```python
from build123d import *

# Parameters (mm, degrees)
SKETCH1_W            = 24
SKETCH1_H            = 24
BOSS_EXTRUDE1_DEPTH  = 3
SKETCH2_W            = 16.6
SKETCH2_H            = 12
BOSS_EXTRUDE2_DEPTH  = 8
CUT_EXTRUDE1_DEPTH   = 21.223748416
CUT_EXTRUDE2_REACH   = 30.26
SKETCH4_R            = 1.6
CUT_EXTRUDE3_DEPTH   = 1.3
FILLET3_R            = 6
CHAMFER3_SIZE        = 3
FILLET4_R            = 3
FILLET6_R            = 1
SKETCH9_R            = 1.6
CUT_EXTRUDE5_DEPTH   = 19.761663039
FILLET8_R            = 3
FILLET9_R            = 0.5
CUT_EXTRUDE6_START   = -1
CUT_EXTRUDE6_DEPTH   = 20.761663103
MIRROR2_START        = -1
MIRROR2_COPY_1_DEPTH = 20.761663103


with BuildPart() as part:
    # Sketch1 → Boss-Extrude1 (new body)
    with BuildSketch(Plane(origin=(0, 0, 0), x_dir=(1, 0, 0), z_dir=(0, 1, 0))):
        Rectangle(SKETCH1_W, SKETCH1_H)
    extrude(amount=BOSS_EXTRUDE1_DEPTH)

    # Sketch2 → Boss-Extrude2 (add)
    with BuildSketch(Plane(origin=(0, 3, 0), x_dir=(1, 0, 0), z_dir=(0, 1, 0))):
        with Locations((-2.8, 0)):
            Rectangle(SKETCH2_W, SKETCH2_H)
    extrude(amount=BOSS_EXTRUDE2_DEPTH)

    # Sketch3 → Cut-Extrude1 (cut, through all)
    with BuildSketch(Plane(origin=(0, 11, 0), x_dir=(1, 0, 0), z_dir=(0, 1, 0))):
        with BuildLine():
            Line((-1.9, 1.774823935), (-1.9, -1.774823935))
            ThreePointArc((-1.9, -1.774823935), (2.6, 0), (-1.9, 1.774823935))
        make_face()
    extrude(amount=-CUT_EXTRUDE1_DEPTH, mode=Mode.SUBTRACT)

    # Sketch4 → Cut-Extrude2 (cut, up to next)
    with BuildSketch(Plane.ZY.offset(11.1), mode=Mode.PRIVATE) as cut_extrude2_sk1:
        with Locations((0, 7)):
            Circle(SKETCH4_R)
    cut_extrude2_tool1 = extrude(cut_extrude2_sk1.sketch, amount=-CUT_EXTRUDE2_REACH, mode=Mode.PRIVATE) & part.part
    add(cut_extrude2_tool1.solids().sort_by_distance((-11.1, 7, 0))[0], mode=Mode.SUBTRACT)

    # Sketch5 → Cut-Extrude3 (cut, symmetric)
    with BuildSketch(Plane(origin=(-4.9, 0, 0), x_dir=(0, 0, -1), z_dir=(1, 0, 0))):
        Polygon((1.645448267, 4.15), (3.290896534, 7), (3.290896534, 11), (-3.290896534, 11), (-3.290896534, 7), (-1.645448267, 4.15), align=None)
    extrude(amount=CUT_EXTRUDE3_DEPTH, both=True, mode=Mode.SUBTRACT)

    # Fillet3
    fillet3_edges = [part.edges().sort_by_distance(p)[0] for p in [
        (5.5, 7, 6),
        (5.5, 7, -6),
    ]]
    fillet(fillet3_edges, radius=FILLET3_R - 0.0001)  # a hair under: the kernel refuses the full size

    # Chamfer3
    chamfer3_edges = [part.edges().sort_by_distance(p)[0] for p in [
        (-11.1, 7, -6),
        (-11.1, 7, 6),
    ]]
    chamfer(chamfer3_edges, length=CHAMFER3_SIZE)

    # Fillet4
    fillet4_edges = [part.edges().sort_by_distance(p)[0] for p in [
        (-8.1, 7, -6),
        (-8.1, 7, 6),
    ]]
    fillet(fillet4_edges, radius=FILLET4_R)

    # Fillet6
    fillet6_edges = [part.edges().sort_by_distance(p)[0] for p in [
        (-3.678629656, 11, -6),
        (3.742669976, 11, -4.242669976),
        (3.742669976, 11, 4.242669976),
        (-3.678629656, 3, -6),
        (3.742669976, 3, 4.242669976),
        (3.742669976, 3, -4.242669976),
        (-10.039339828, 11, 4.060660172),
        (-10.039339828, 3, -4.060660172),
        (-3.678629656, 11, 6),
        (-3.678629656, 3, 6),
        (-10.039339828, 3, 4.060660172),
        (-10.039339828, 11, -4.060660172),
        (-8.00540961, 11, -5.771638598),
        (-8.00540961, 11, 5.771638598),
        (-8.00540961, 3, 5.771638598),
        (-8.00540961, 3, -5.771638598),
    ]]
    fillet(fillet6_edges, radius=FILLET6_R)

    # Sketch9 → Cut-Extrude5 (cut, through all)
    with BuildSketch(Plane(origin=(0, 3, 0), x_dir=(1, 0, 0), z_dir=(0, 1, 0))):
        with Locations(Location((-9, 9, 0), (0, 0, 270))):
            Circle(SKETCH9_R)
        with Locations(Location((9, 9, 0), (0, 0, 270))):
            Circle(SKETCH9_R)
        with Locations(Location((9, -9, 0), (0, 0, 270))):
            Circle(SKETCH9_R)
        with Locations(Location((-9, -9, 0), (0, 0, 270))):
            Circle(SKETCH9_R)
    extrude(amount=-CUT_EXTRUDE5_DEPTH, mode=Mode.SUBTRACT)

    # Fillet8
    fillet8_edges = [part.edges().sort_by_distance(p)[0] for p in [
        (-12, 1.5, -12),
        (12, 1.5, -12),
        (12, 1.5, 12),
        (-12, 1.5, 12),
    ]]
    fillet(fillet8_edges, radius=FILLET8_R)

    # Fillet9
    fillet9_edges = [part.edges().sort_by_distance(p)[0] for p in [
        (12, 3, 0),
        (0, 3, 12),
        (-12, 3, 0),
        (0, 3, -12),
        (-11.121320344, 3, 11.121320344),
        (-11.121320344, 3, -11.121320344),
        (11.121320344, 3, -11.121320344),
        (11.121320344, 3, 11.121320344),
    ]]
    fillet(fillet9_edges, radius=FILLET9_R)

    # Sketch10 → Cut-Extrude6 (cut)
    with BuildSketch(Plane(origin=(0, 3, 0), x_dir=(1, 0, 0), z_dir=(0, 1, 0)).offset(CUT_EXTRUDE6_START)):
        Polygon((5.821238046, -9.851746699), (8.148253301, -12.178761954), (9.106066017, -13.13657467), (13.13657467, -9.106066017), (12.178761954, -8.148253301), (9.851746699, -5.821238046), (6.672984744, -6.672984744), align=None)
    cut_extrude6 = extrude(amount=CUT_EXTRUDE6_DEPTH, mode=Mode.SUBTRACT)

    # Mirror1: Cut-Extrude6 across plane
    add(cut_extrude6.mirror(Plane.XY), mode=Mode.SUBTRACT)

    # Mirror2: Cut-Extrude6 across plane
    add(cut_extrude6.mirror(Plane(origin=(0, 0, 0), x_dir=(0, 0, 1), z_dir=(1, 0, 0))), mode=Mode.SUBTRACT)

    # Mirror2 copy 1 sketch → Mirror2 copy 1 (cut)
    with BuildSketch(Plane(origin=(0, 3, 0), x_dir=(-1, 0, 0), z_dir=(0, 1, 0)).offset(MIRROR2_START)):
        Polygon((5.821238046, -9.851746699), (8.148253301, -12.178761954), (9.106066017, -13.13657467), (13.13657467, -9.106066017), (12.178761954, -8.148253301), (9.851746699, -5.821238046), (6.672984744, -6.672984744), align=None)
    extrude(amount=MIRROR2_COPY_1_DEPTH, mode=Mode.SUBTRACT)


solid = part.part
```
Here's how the part is built. I have some questions about the finished solid (model axes, mm). A direction names the side the tool comes from. Round coordinates to 2 decimals unless told otherwise and drop trailing zeros. Order: outer loops, then holes, each group sorted by start corner. A loop starts at its lowest first (then second) coordinate and runs counter-clockwise, first axis right, second up. Notation, with made-up numbers: (34.5, 85.5) -> (66.5, 85.5) arc R15 cw to (66.5, 95.5) -> close; hole circle Ø1 at (-23.5, 33). An arc over 180 degrees is marked (long way). Use a Markdown table: item, result. Add a question column.
(1) Suppose I cut it at D-D, the plane y = 5. Count the separate pieces of the cut face and the enclosed holes in it, and give its area (3 significant figures).
(2) I need wall thicknesses on line 1 along X through (y, z) = (4.25, 0); line 2 along X through (y, z) = (1.25, -9); line 3 along Z through (x, y) = (9.5, 0.5). Which ranges of each line are inside material? Lowest first, please.
(3) If we mould it in two halves opening along Z, with no side actions, what happens to faces 1 (the face through (10, 2, 7)), 2 (the face through (-4, 7, -6)), 3 (the face through (-10.94, 2.49, 6.91)), 4 (the face through (-8.285, 2.559, -6.241))? For each: released by +Z, released by -Z, zero draft, split by the parting line, or undercut.
(4) For faces 5 (the face through (-10, 7, -4.1)), 6 (the face through (-4, 7, 6)), 7 (the face through (-10.94, 2.49, -6.91)), 8 (the face through (-4.88, 5.56, -2.46)), 9 (the face through (-6.88, 2.49, 10.91)), which set-ups out of +Z, -Z, +X, -X, +Y, -Y let a thin tool reach every point of the face, with its end or its side?
(5) For pin 1 Ø1.9 at (x, z) = (-7.5, -8.5) entering from +Y; pin 2 Ø1.1 at (y, z) = (8, 0) entering from +X; pin 3 Ø1.9 at (y, z) = (7, 0) entering from -X, each with a flat end and sliding along its axis, tell me the tip position at first contact or that it passes through.
(6) Suppose I cut it at B-B, the plane x = -4.5. Please give me the cut outline in (y, z), and give its area (3 significant figures).
(7) Suppose I cut it at A-A, the plane y = 1. Please give me the cut outline in (x, z).
(8) Suppose I cut it at C-C, the plane x = 8.5. Please give me the cut outline in (y, z), and give its area (3 significant figures).
Verdict:
| question | item | result |
|---|---|---|
| 1 | separate pieces | 1 |
| 1 | enclosed holes | 2 |
| 1 | area | 144 mm2 |
| 2 | line 1 | -11.1 to -6.2, -3.6 to -1.9, 2.6 to 5.5 |
| 2 | line 2 | -12 to -10.6, -7.4 to 7.4, 10.6 to 12 |
| 2 | line 3 | -11.96 to -10.52, -7.48 to 7.48, 10.52 to 11.96 |
| 3 | face 1 | undercut |
| 3 | face 2 | released by -Z |
| 3 | face 3 | released by +Z |
| 3 | face 4 | undercut |
| 4 | face 5 | -Z, -X, +Y |
| 4 | face 6 | +Z, +X, -X, +Y |
| 4 | face 7 | -Z, +Y |
| 4 | face 8 | +Y |
| 4 | face 9 | -X, +Y |
| 5 | pin 1 | y = 2 |
| 5 | pin 2 | x = 5.5 |
| 5 | pin 3 | x = 2.42 |
| 6 | outline | (0, -12) -> (2.5, -12) arc R0.5 ccw to (3, -11.5) -> (3, -7) arc R1 cw to (4, -6) -> (10, -6) arc R1 ccw to (11, -5) -> (11, -3.29) -> (7, -3.29) -> (4.15, -1.65) -> (4.15, 1.65) -> (7, 3.29) -> (11, 3.29) -> (11, 5) arc R1 ccw to (10, 6) -> (4, 6) arc R1 cw to (3, 7) -> (3, 11.5) arc R0.5 ccw to (2.5, 12) -> (0, 12) -> close |
| 6 | area | 127 mm2 |
| 7 | outline | (-12, -9) arc R3 ccw to (-9, -12) -> (9, -12) arc R3 ccw to (12, -9) -> (12, 9) arc R3 ccw to (9, 12) -> (-9, 12) arc R3 ccw to (-12, 9) -> close; hole circle Ø3.2 at (-9, -9); hole circle Ø3.2 at (-9, 9); hole (-1.9, -1.77) arc R2.6 ccw (long way) to (-1.9, 1.77) -> close; hole circle Ø3.2 at (9, -9); hole circle Ø3.2 at (9, 9) |
| 8 | outline | (0, -12) -> (2, -12) -> (2, -10.52) -> (0, -10.52) -> close; (0, -7.48) -> (2, -7.48) -> (2, -6.18) -> (3, -6.18) -> (3, 6.18) -> (2, 6.18) -> (2, 7.48) -> (0, 7.48) -> close; (0, 10.52) -> (2, 10.52) -> (2, 12) -> (0, 12) -> close |
| 8 | area | 48.2 mm2 |
